Geometry check sheet. Reference: the model listing, model coordinates, mm. Face numbers are marked on the shaded views. A direction names the side the tool comes from. Give positions to 0.01 mm unless a question says otherwise; leave off trailing zeros. Loops run counter-clockwise (first coordinate to the right, second up) from the corner with the lowest first, then second, coordinate; pieces in that order, holes last. Notation, with made-up numbers: (51, -19.5) -> (101, -19.5) arc R15 cw to (101, -3.5) -> close; hole circle Ø4 at (-36.75, -35). An arc over 180 degrees is marked (long way). Answer as a JSON object with one key per item and string values.
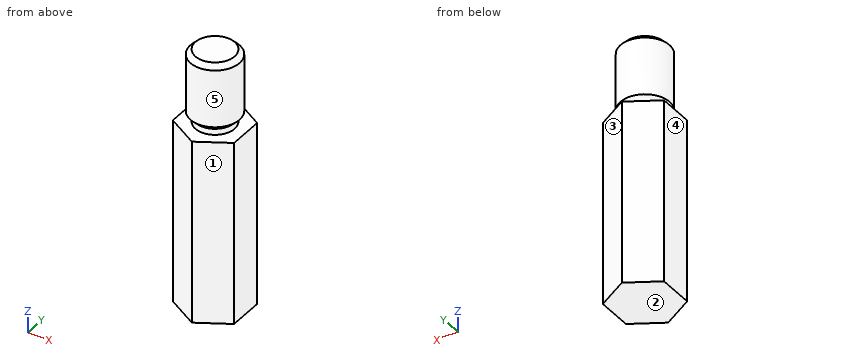
from build123d import *

# Parameters (mm, degrees)
EXTRUDE_1_DEPTH     = 15
SKETCH_2_R          = 2
EXTRUDE_2_DEPTH     = 6
SKETCH_3_R          = 2
SKETCH_3_R_2        = 1.6
CUT_EXTRUDE_3_DEPTH = 0.5
CHAMFER_1_SIZE      = 0.4


with BuildPart() as part:
    # Эскиз1 → Вытянуть1 (new body)
    with BuildSketch(Plane.XY):
        Polygon((0, 2.886751346), (-2.5, 1.443375673), (-2.5, -1.443375673), (0, -2.886751346), (2.5, -1.443375673), (2.5, 1.443375673), align=None)
    extrude(amount=EXTRUDE_1_DEPTH)

    # Эскиз2 → Вытянуть2 (add)
    with BuildSketch(Plane.XY.offset(15)):
        Circle(SKETCH_2_R)
    extrude(amount=EXTRUDE_2_DEPTH)

    # Эскиз3 → Вырез-Вытянуть3 (cut)
    with BuildSketch(Plane.XY.offset(15)):
        Circle(SKETCH_3_R)
        Circle(SKETCH_3_R_2, mode=Mode.SUBTRACT)
    extrude(amount=CUT_EXTRUDE_3_DEPTH, mode=Mode.SUBTRACT)

    # Фаска1
    chamfer_1_edges = [part.edges().sort_by_distance(p)[0] for p in [
        (-2, 0, 21),
        (-2, 0, 15.5),
    ]]
    chamfer(chamfer_1_edges, length=CHAMFER_1_SIZE - 0.0001)  # a hair under: the kernel refuses the full size


solid = part.part
1) Depth check by flat-ended pin: P1, Ø1, axis at y = -1.5, z = 17.5, coming from the +X side. Enter the tip coordinate at first touch or a pass-through.
Geometry check:
{"P1": "stops at x = 1.73"}
2) Draft check along Y on the marked faces 1, 2 and 3. Enter one of: pulls with the +Y half, pulls with the -Y half, needs draft (parallel to the pull), parting line crosses it, or undercut.
Geometry check:
{"face 1": "pulls with the -Y half", "face 2": "needs draft", "face 3": "pulls with the +Y half"}
3) Section check B-B on z = 6.75. Record the cut outline in (x, y), plus the area to 3 significant figures.
Geometry check:
{"outline": "(-2.5, -1.44) -> (0, -2.89) -> (2.5, -1.44) -> (2.5, 1.44) -> (0, 2.89) -> (-2.5, 1.44) -> close", "area": "21.7 mm2"}
4) Tool access check on the marked faces 4 and 5. Record the directions out of +Z, -Z, +X, -X, +Y, -Y that give a thin tool (end or side, any length) a straight path to the whole face; none if there is none.
Geometry check:
{"face 4": "+Z, -Z, -X, +Y, -Y", "face 5": "+Z"}
5) Section check C-C on z = 18.5. Record the cut outline in (x, y), plus the area to 3 significant figures.
Geometry check:
{"outline": "circle Ø4 at (0, 0)", "area": "12.6 mm2"}
6) Material ranges on line 1 along Z through (x, y) = (1.2, -1.35); line 2 along Z through (x, y) = (-0.7, -2.2); line 3 along Z through (x, y) = (-1.6, -0.6), recorded low to high. Write a range as from..to.
Geometry check:
{"line 1": "z = 0..15, 15.71..20.79", "line 2": "z = 0..15", "line 3": "z = 0..15, 15.61..20.89"}
